from build123d import *

# Parameters (mm, degrees)
F0_W     = 62
F0_H     = 62
F0_R     = 20.75
F1_DEPTH = 53
F2_R     = 23.75
F2_R_2   = 20.75
F3_DEPTH = 4
F4_R     = 27.5
F4_R_2   = 20.75
F5_DEPTH = 5
F7_DEPTH = 53.001


with BuildPart() as f1:
    # F0 (on Top) → F1 (new body)
    with BuildSketch(Plane.XY):
        Rectangle(F0_W, F0_H)
        Circle(F0_R, mode=Mode.SUBTRACT)
    extrude(amount=F1_DEPTH)

    # F2 (on face) → F3 (join)
    with BuildSketch(Plane.XY.offset(53)):
        Circle(F2_R)
        Circle(F2_R_2, mode=Mode.SUBTRACT)
    extrude(amount=F3_DEPTH)

    # F4 (on face) → F5 (cut)
    with BuildSketch(Plane(origin=(0, 0, 0), x_dir=(1, 0, 0), z_dir=(0, 0, -1))):
        Circle(F4_R)
        Circle(F4_R_2, mode=Mode.SUBTRACT)
    extrude(amount=-F5_DEPTH, mode=Mode.SUBTRACT)

    # F6 (on face) → F7 (cut, through all)
    with BuildSketch(Plane.XY.offset(53)):
        with BuildLine():
            ThreePointArc((-24.679438301, 21.1465204028), (-22.9809703886, 22.9809703886), (-21.1465204028, 24.679438301))
            ThreePointArc((-21.1465204028, 24.679438301), (-24.7487373415, 24.7487373415), (-24.679438301, 21.1465204028))
        make_face()
        with BuildLine():
            ThreePointArc((-20.4809703886, 22.9809703886), (-20.653297198, 23.8930764777), (-21.1465204028, 24.679438301))
            ThreePointArc((-21.1465204028, 24.679438301), (-22.9809703886, 22.9809703886), (-24.679438301, 21.1465204028))
            ThreePointArc((-24.679438301, 21.1465204028), (-21.9800132919, 20.6901004903), (-20.4809703886, 22.9809703886))
        make_face()
        with BuildLine():
            ThreePointArc((21.1465204028, 24.679438301), (22.0800828621, 23.8478498151), (22.9809703886, 22.9809703886))
            Line((22.9809703886, 22.9809703886), (24.7487373415, 24.7487373415))
            ThreePointArc((24.7487373415, 24.7487373415), (22.9328845698, 25.4805078966), (21.1465204028, 24.679438301))
        make_face()
        with BuildLine():
            ThreePointArc((22.9809703886, 22.9809703886), (23.8478498151, 22.0800828621), (24.679438301, 21.1465204028))
            ThreePointArc((24.679438301, 21.1465204028), (25.2718402868, 21.9800132919), (25.4809703886, 22.9809703886))
            ThreePointArc((25.4809703886, 22.9809703886), (25.2906692198, 23.9376789695), (24.7487373415, 24.7487373415))
            Line((24.7487373415, 24.7487373415), (22.9809703886, 22.9809703886))
        make_face()
        with BuildLine():
            ThreePointArc((21.2132034356, 21.2132034356), (22.9328845698, 20.4814328805), (24.679438301, 21.1465204028))
            ThreePointArc((24.679438301, 21.1465204028), (23.8478498151, 22.0800828621), (22.9809703886, 22.9809703886))
            Line((22.9809703886, 22.9809703886), (21.2132034356, 21.2132034356))
        make_face()
        with BuildLine():
            Line((21.2132034356, 21.2132034356), (22.9809703886, 22.9809703886))
            ThreePointArc((22.9809703886, 22.9809703886), (22.0800828621, 23.8478498151), (21.1465204028, 24.679438301))
            ThreePointArc((21.1465204028, 24.679438301), (20.4814328805, 22.9328845698), (21.2132034356, 21.2132034356))
        make_face()
        with BuildLine():
            ThreePointArc((21.1465204028, -24.679438301), (22.9809703886, -22.9809703886), (24.679438301, -21.1465204028))
            ThreePointArc((24.679438301, -21.1465204028), (21.2132034356, -21.2132034356), (21.1465204028, -24.679438301))
        make_face()
        with BuildLine():
            ThreePointArc((25.4809703886, -22.9809703886), (25.2718402868, -21.9800132919), (24.679438301, -21.1465204028))
            ThreePointArc((24.679438301, -21.1465204028), (22.9809703886, -22.9809703886), (21.1465204028, -24.679438301))
            ThreePointArc((21.1465204028, -24.679438301), (23.8930764777, -25.3086435792), (25.4809703886, -22.9809703886))
        make_face()
        with BuildLine():
            ThreePointArc((-24.679438301, -21.1465204028), (-24.7487373415, -24.7487373415), (-21.1465204028, -24.679438301))
            ThreePointArc((-21.1465204028, -24.679438301), (-22.9809703886, -22.9809703886), (-24.679438301, -21.1465204028))
        make_face()
        with BuildLine():
            ThreePointArc((-24.679438301, -21.1465204028), (-22.9809703886, -22.9809703886), (-21.1465204028, -24.679438301))
            ThreePointArc((-21.1465204028, -24.679438301), (-20.653297198, -23.8930764777), (-20.4809703886, -22.9809703886))
            ThreePointArc((-20.4809703886, -22.9809703886), (-21.9800132919, -20.6901004903), (-24.679438301, -21.1465204028))
        make_face()
    extrude(amount=-F7_DEPTH, mode=Mode.SUBTRACT)


solid = f1.part
Verification items for the finished model (mm, model axes). A direction names the side the tool comes from. Coordinates: 2 decimals unless noted, no trailing zeros. Write each loop counter-clockwise with the first axis right and the second up, starting at its lowest first coordinate (ties: lowest second). Pieces come first, ordered by that corner, then holes. Notation, with made-up numbers: M -32.75,-7 L -21.75,-7 A19 ccw -21.75,21 Z; hole C 21.25,-32.75 d10. An arc over 180 degrees is marked long. One line per question, with ' | ' between items.
1) Sectioned sample at A-A on y = 0. Record the cut outline in (x, z).
Solutions:
outline: M -31,0 L -27.5,0 L -27.5,5 L -20.75,5 L -20.75,57 L -23.75,57 L -23.75,53 L -31,53 Z; M 20.75,5 L 27.5,5 L 27.5,0 L 31,0 L 31,53 L 23.75,53 L 23.75,57 L 20.75,57 Z
2) Access from +Z, -Z, +X, -X, +Y, -Y to the whole of each face (thin tool, end or side, straight path). Record for faces 4 (the face through (0, -21, 57)), 5 (the face through (-5.961, 26.846, 2.465)), 6 (the face through (-14, 21, 53)).
Solutions:
face 4: +Z, +X, -X, +Y, -Y | face 5: -Z | face 6: +Z
3) Material ranges on L1, parallel to X at y = 0, z = 20.5; L2, parallel to Y at x = 0, z = 1.2, recorded low to high.
Solutions:
L1: -31 to -20.75, 20.75 to 31 | L2: -31 to -27.5, 27.5 to 31
4) Sectioned sample at C-C on z = 6. Record the cut outline in (x, y), then the cut area to 3 significant figures.
Solutions:
outline: M -31,-31 L 31,-31 L 31,31 L -31,31 Z; hole C -22.98,-22.98 d5; hole C -22.98,22.98 d5; hole C 0,0 d41.5; hole C 22.98,-22.98 d5; hole C 22.98,22.98 d5 | area: 2,410 mm^2
5) Release check for a two-part mould opening along Y. For faces 1 (the face through (-31, 0, 26)), 2 (the face through (-10.3, -18.5, 5)), 3 (the face through (-5.149, -23.185, 54.972)) record: +Y half, -Y half, draft (parallel to the pull), parting line (faces both ways), or undercut.
Solutions:
face 1: draft | face 2: undercut | face 3: parting line
6) Depth check by flat-ended pin: pin 1 Ø25 at (x, y) = (0, 0) entering from -Z; pin 2 Ø6 at (x, y) = (18, -21) entering from -Z. Enter the tip coordinate at first touch or a pass-through.
Solutions:
pin 1: through | pin 2: z = 0
